Source: three-view drawing plus pictorial views. Frame: mm from the lowest corner of the part. Give positions to 0.01 mm unless a question says otherwise; leave off trailing zeros. Order: outer loops, then holes, each group sorted by start corner. A loop starts at its lowest first (then second) coordinate and runs counter-clockwise, first axis right, second up.
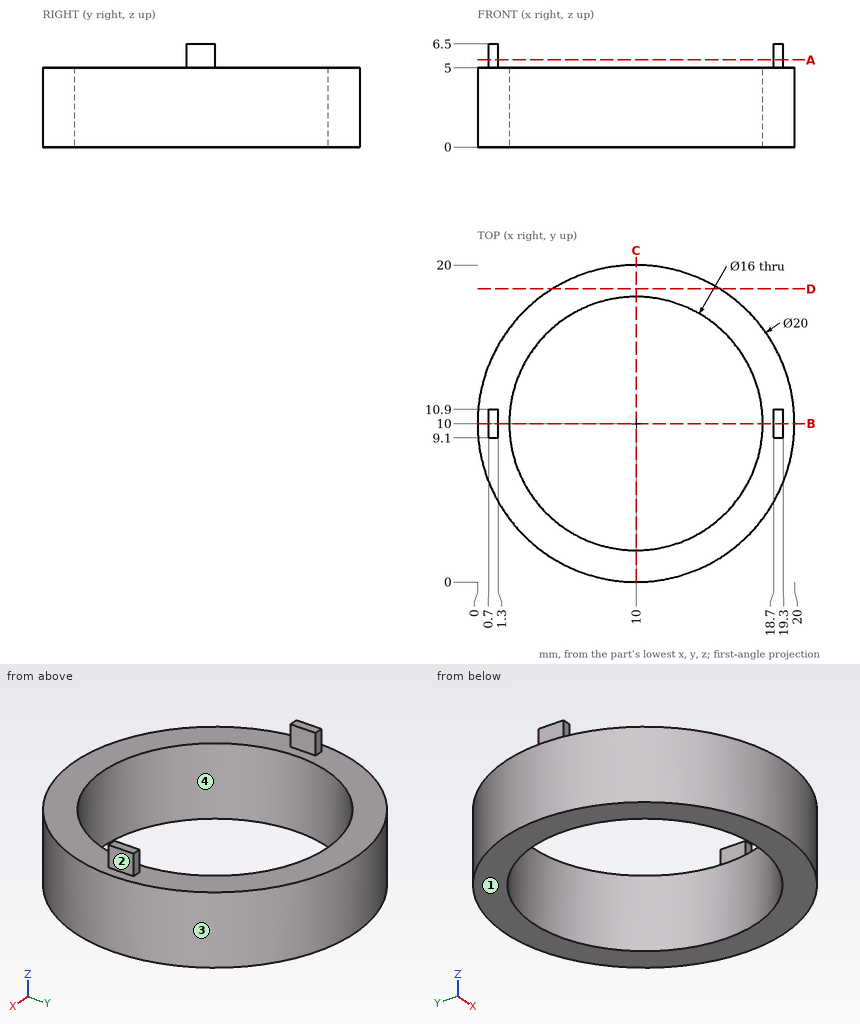
(1) Section B-B, the plane y = 10. Return loops of the section in (x, z), plus the area to 3 significant figures.
(2) Pin query (flat end, axial travel): pin 1 Ø12 at (x, y) = (2, 8.5) entering from +Z; pin 2 Ø6 at (x, y) = (8, 13) entering from +Z; pin 3 Ø0.7 at (x, z) = (19, 5.5) entering from +Y; pin 4 Ø0.8 at (y, z) = (9.5, 5.5) entering from +X. Return the tip coordinate at first contact, or that it passes through.
(3) Section A-A, the plane z = 5.5. Return loops of the section in (x, y).
(4) Section D-D, the plane y = 18.5. Return loops of the section in (x, z), plus the area to 3 significant figures.
(5) Section C-C, the plane x = 10. Return loops of the section in (y, z).
(6) Line query: line 1 along Y through (x, z) = (10, 2.8); line 2 along Z through (x, y) = (10, 1); line 3 along Y through (x, z) = (12.25, 1.25). Output: solid intervals per line, ascending.
(7) Draft query along X for the marked faces 1, 2, 3 and 4. Return one class per face: +X half, -X half, draft (parallel to the pull), parting line (faces both ways), or undercut.
Checks:
1. outline: (0, 0) - (2, 0) - (2, 5) - (1.3, 5) - (1.3, 6.5) - (0.7, 6.5) - (0.7, 5) - (0, 5) - close; (18, 0) - (20, 0) - (20, 5) - (19.3, 5) - (19.3, 6.5) - (18.7, 6.5) - (18.7, 5) - (18, 5) - close
1. area: 21.8 mm2
2. pin 1: stops at z = 6.5
2. pin 2: passes through
2. pin 3: stops at y = 10.9
2. pin 4: stops at x = 19.3
3. outline: (0.7, 9.1) - (1.3, 9.1) - (1.3, 10.9) - (0.7, 10.9) - close; (18.7, 9.1) - (19.3, 9.1) - (19.3, 10.9) - (18.7, 10.9) - close
4. outline: (4.73, 0) - (15.27, 0) - (15.27, 5) - (4.73, 5) - close
4. area: 52.7 mm2
5. outline: (0, 0) - (2, 0) - (2, 5) - (0, 5) - close; (18, 0) - (20, 0) - (20, 5) - (18, 5) - close
6. line 1: y = 0 to 2, 18 to 20
6. line 2: z = 0 to 5
6. line 3: y = 0.26 to 2.32, 17.68 to 19.74
7. face 1: draft
7. face 2: +X half
7. face 3: parting line
7. face 4: undercut
